Could you check a few things on this drawing? It's one solid part, dimensions in mm from its lowest x, y, z. Give positions to 0.01 mm unless a question says otherwise; leave off trailing zeros. Order: outer loops, then holes, each group sorted by start corner. A loop starts at its lowest first (then second) coordinate and runs counter-clockwise, first axis right, second up. Notation, with made-up numbers: (81.25, -30) -> (99.25, -30) arc R30 ccw to (99.25, 7) -> close; hole circle Ø6 at (-27, 47). An arc over 180 degrees is marked (long way). Answer as CSV lines item,"result".
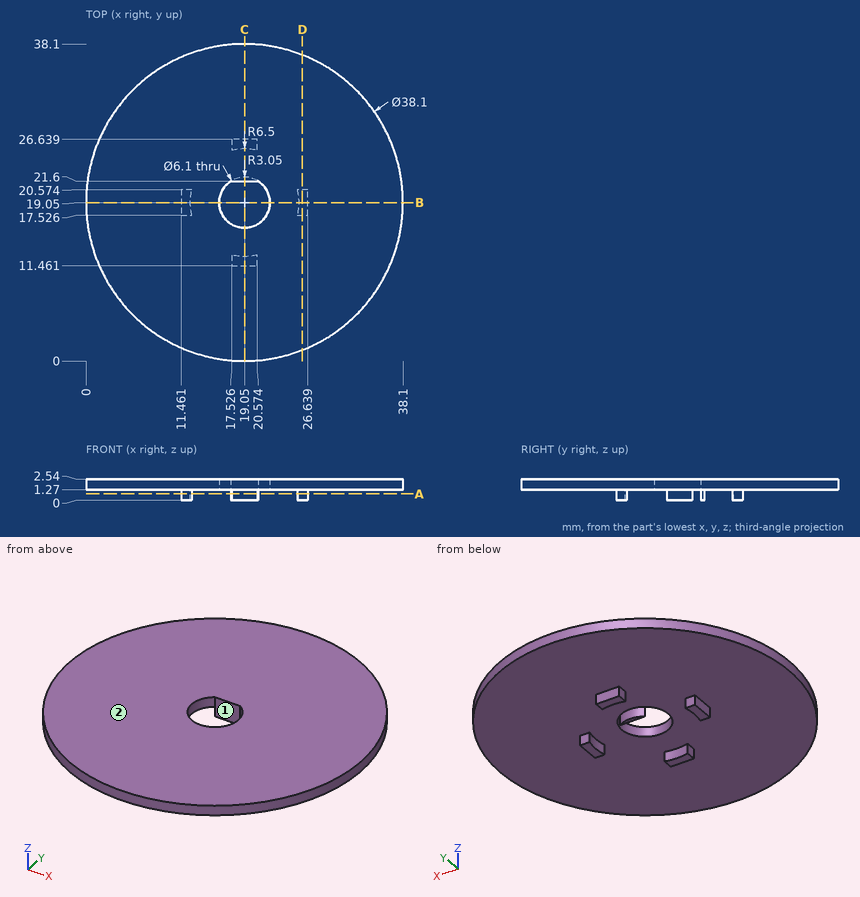
Item 1: Please list where these lines run through material, in increasing order: line 1 along Y through (x, z) = (19.05, 2.2); line 2 along Y through (x, z) = (20, 0.7); line 3 along Z through (x, y) = (15.5, 27).
Numbers:
line 1,"y = 0 to 16, 21.6 to 38.1"
line 2,"y = 11.46 to 12.62, 21.6 to 21.95, 25.48 to 26.64"
line 3,"z = 1.27 to 2.54"
Item 2: Imagine slicing it at D-D, the plane x = 26. Please give me the cut outline in (y, z).
Numbers:
outline,"(1.31, 1.27) -> (17.53, 1.27) -> (17.53, 0) -> (20.57, 0) -> (20.57, 1.27) -> (36.79, 1.27) -> (36.79, 2.54) -> (1.31, 2.54) -> close"
Item 3: Imagine slicing it at B-B, the plane y = 19.05. Please give me the cut outline in (x, z), then the cut area to 3 significant figures.
Numbers:
outline,"(0, 1.27) -> (11.46, 1.27) -> (11.46, 0) -> (12.55, 0) -> (12.55, 1.27) -> (16, 1.27) -> (16, 2.54) -> (0, 2.54) -> close; (22.1, 1.27) -> (25.55, 1.27) -> (25.55, 0) -> (26.64, 0) -> (26.64, 1.27) -> (38.1, 1.27) -> (38.1, 2.54) -> (22.1, 2.54) -> close"
area,"43.4 mm²"
Item 4: Imagine slicing it at C-C, the plane x = 19.05. Please give me the cut outline in (y, z).
Numbers:
outline,"(0, 1.27) -> (11.46, 1.27) -> (11.46, 0) -> (12.55, 0) -> (12.55, 1.27) -> (16, 1.27) -> (16, 2.54) -> (0, 2.54) -> close; (21.6, 0) -> (22.1, 0) -> (22.1, 1.27) -> (25.55, 1.27) -> (25.55, 0) -> (26.64, 0) -> (26.64, 1.27) -> (38.1, 1.27) -> (38.1, 2.54) -> (21.6, 2.54) -> close"
Item 5: We'd pull the mould along Y, two halves only. Please class the marked faces 1 and 2: released by +Y, released by -Y, zero draft, split by the parting line, or undercut.
Numbers:
face 1,"undercut"
face 2,"zero draft"
Item 6: Imagine slicing it at A-A, the plane z = 0.75. Please give me the cut outline in (x, y).
Numbers:
outline,"(11.46, 17.53) -> (12.73, 17.53) arc R6.5 cw to (12.73, 20.57) -> (11.46, 20.57) -> close; (17.38, 21.6) -> (20.72, 21.6) arc R3.05 ccw to start; (17.53, 11.46) -> (20.57, 11.46) -> (20.57, 12.73) arc R6.5 cw to (17.53, 12.73) -> close; (17.53, 25.37) arc R6.5 cw to (20.57, 25.37) -> (20.57, 26.64) -> (17.53, 26.64) -> close; (25.37, 17.53) -> (26.64, 17.53) -> (26.64, 20.57) -> (25.37, 20.57) arc R6.5 cw to start"
Item 7: For pin 1 (1.4 mm diameter, centred on x = 12.5, z = 0.5, fed in from -Y); pin 2 (8 mm diameter, centred on x = 19.05, y = 19.05, fed in from +Z); pin 3 (1 mm diameter, centred on y = 26.5, z = 0.5, fed in from +X); pin 4 (0.6 mm diameter, centred on y = 19, z = 0.5, fed in from -X), each with a flat end and sliding along its axis, tell me the tip position at first contact or that it passes through.
Numbers:
pin 1,"stops at y = 17.53"
pin 2,"stops at z = 2.54"
pin 3,"stops at x = 20.57"
pin 4,"stops at x = 11.46"
